from build123d import *

# Parameters (mm, degrees)
F0_W     = 58
F0_H     = 36
F0_R     = 1.25
F0_R_2   = 1.5
F1_DEPTH = 10
F0_R_3   = 1
F0_W_2   = 3.2825097442
F0_H_2   = 9.0816104785
F0_R_4   = 4
F2_DEPTH = 2.5
F3_R     = 3
F4_DEPTH = 6
F5_START = 0.9
F5_DEPTH = 16.2
F6_START = 6
F6_DEPTH = 10.7
F7_R     = 1


with BuildPart() as f1:
    # F0 (on Top) → F1 (new body)
    with BuildSketch(Plane.XY):
        with Locations((22.1260370687, 12.181818096)):
            Rectangle(F0_W, F0_H)
        with Locations((-2.8739629313, -1.818181904)):
            Circle(F0_R, mode=Mode.SUBTRACT)
        with Locations((3.1260370687, -3.018181904)):
            Circle(F0_R_2, mode=Mode.SUBTRACT)
        with Locations((41.1260370687, -3.018181904)):
            Circle(F0_R_2, mode=Mode.SUBTRACT)
        with Locations((47.1260370687, -1.818181904)):
            Circle(F0_R, mode=Mode.SUBTRACT)
        with BuildLine():
            Line((-0.0042433119, 0.0237876128), (-0.0123524841, 0.02397218))
            Line((-0.0123524841, 0.02397218), (-0.0123524841, 0.0693824727))
            ThreePointArc((-0.0123524841, 0.0693824727), (-1.0671188126, 12.0466773263), (-0.0123524841, 24.02397218))
            ThreePointArc((-0.0123524841, 24.02397218), (22.4498159336, 26.0118318189), (44.9770614896, 25))
            ThreePointArc((44.9770614896, 25), (46.474513746, 12), (44.9770614896, -1))
            ThreePointArc((44.9770614896, -1), (22.4574664967, -1.8971785964), (0, 0))
            ThreePointArc((0, 0), (-0.0021227043, 0.0118936194), (-0.0042433119, 0.0237876128))
        make_face(mode=Mode.SUBTRACT)
        with Locations((-2.8739629313, 26.181818096)):
            Circle(F0_R, mode=Mode.SUBTRACT)
        with Locations((3.1260370687, 27.16396598)):
            Circle(F0_R_2, mode=Mode.SUBTRACT)
        with Locations((41.1260370687, 27.6376707083)):
            Circle(F0_R_2, mode=Mode.SUBTRACT)
        with Locations((47.1260370687, 26.181818096)):
            Circle(F0_R, mode=Mode.SUBTRACT)
        with Locations((-2.8739629313, 26.181818096)):
            Circle(F0_R)
        with Locations((47.1260370687, 26.181818096)):
            Circle(F0_R)
        with Locations((47.1260370687, -1.818181904)):
            Circle(F0_R)
        with Locations((-2.8739629313, -1.818181904)):
            Circle(F0_R)
        with Locations((3.1260370687, -3.018181904)):
            Circle(F0_R_2)
        with Locations((3.1260370687, 27.16396598)):
            Circle(F0_R_2)
        with Locations((41.1260370687, 27.6376707083)):
            Circle(F0_R_2)
        with Locations((41.1260370687, -3.018181904)):
            Circle(F0_R_2)
    extrude(amount=F1_DEPTH)

    # F0 (on Top) → F2 (join)
    with BuildSketch(Plane.XY):
        with BuildLine():
            ThreePointArc((-0.0123524841, 24.02397218), (-1.0671188126, 12.0466773263), (-0.0123524841, 0.0693824727))
            Line((-0.0123524841, 0.0693824727), (-0.0123524841, 24.02397218))
        make_face()
        with BuildLine():
            Line((-0.0123524841, 24.02397218), (-0.0123524841, 0.0693824727))
            ThreePointArc((-0.0123524841, 0.0693824727), (-0.0083017494, 0.0465843578), (-0.0042433119, 0.0237876128))
            Line((-0.0042433119, 0.0237876128), (44.9770614896, -1))
            Line((44.9770614896, -1), (44.9770614896, 25))
            Line((44.9770614896, 25), (-0.0123524841, 24.02397218))
        make_face()
        with Locations((2.9621722015, 2.0848012064)):
            Circle(F0_R_3, mode=Mode.SUBTRACT)
        with Locations((5.0146379508, 11.9371688925)):
            Rectangle(F0_W_2, F0_H_2, mode=Mode.SUBTRACT)
        with Locations((41.7125664489, 2.0848012064)):
            Circle(F0_R_3, mode=Mode.SUBTRACT)
        with BuildLine():
            Line((26.1260370687, 7.1930042468), (26.1260370687, 9.181818096))
            Line((26.1260370687, 9.181818096), (26.4652403515, 9.181818096))
            ThreePointArc((26.4652403515, 9.181818096), (32.1260370687, 13.1930042468), (37.7868337859, 9.181818096))
            Line((37.7868337859, 9.181818096), (38.1260370687, 9.181818096))
            Line((38.1260370687, 9.181818096), (38.1260370687, 7.1930042468))
            Line((38.1260370687, 7.1930042468), (38.1260370687, 1.181818096))
            Line((38.1260370687, 1.181818096), (26.1260370687, 1.181818096))
            Line((26.1260370687, 1.181818096), (26.1260370687, 7.1930042468))
        make_face(mode=Mode.SUBTRACT)
        with Locations((41.1260370687, 12.181818096)):
            Circle(F0_R_2, mode=Mode.SUBTRACT)
        with Locations((18.8074270263, 12.2937392443)):
            Circle(F0_R_3, mode=Mode.SUBTRACT)
        with Locations((2.9621722015, 21.6664075851)):
            Circle(F0_R_3, mode=Mode.SUBTRACT)
        with Locations((26.8074270263, 12.2937392443)):
            Circle(F0_R_3, mode=Mode.SUBTRACT)
        with Locations((32.1260370687, 19.181818096)):
            Circle(F0_R_4, mode=Mode.SUBTRACT)
        with Locations((41.7125664489, 21.6664075851)):
            Circle(F0_R_3, mode=Mode.SUBTRACT)
        with BuildLine():
            Line((44.9770614896, -1), (-0.0042433119, 0.0237876128))
            ThreePointArc((-0.0042433119, 0.0237876128), (-0.0021227043, 0.0118936194), (0, 0))
            ThreePointArc((0, 0), (22.4574664967, -1.8971785964), (44.9770614896, -1))
        make_face()
        with BuildLine():
            ThreePointArc((44.9770614896, 25), (22.4498159336, 26.0118318189), (-0.0123524841, 24.02397218))
            Line((-0.0123524841, 24.02397218), (44.9770614896, 25))
        make_face()
        with BuildLine():
            Line((44.9770614896, 25), (44.9770614896, -1))
            ThreePointArc((44.9770614896, -1), (46.474513746, 12), (44.9770614896, 25))
        make_face()
        with Locations((2.9621722015, 21.6664075851)):
            Circle(F0_R_3)
        with Locations((2.9621722015, 2.0848012064)):
            Circle(F0_R_3)
        with Locations((41.7125664489, 2.0848012064)):
            Circle(F0_R_3)
        with Locations((41.7125664489, 21.6664075851)):
            Circle(F0_R_3)
        with Locations((18.8074270263, 12.2937392443)):
            Circle(F0_R_3)
        with Locations((26.8074270263, 12.2937392443)):
            Circle(F0_R_3)
        with Locations((5.0146379508, 11.9371688925)):
            Rectangle(F0_W_2, F0_H_2)
        with BuildLine():
            Line((26.4652403515, 9.181818096), (26.1260370687, 9.181818096))
            Line((26.1260370687, 9.181818096), (26.1260370687, 7.1930042468))
            ThreePointArc((26.1260370687, 7.1930042468), (26.2114457767, 8.2017707453), (26.4652403515, 9.181818096))
        make_face()
        with BuildLine():
            ThreePointArc((38.1260370687, 7.1930042468), (32.1260370687, 1.1930042468), (26.1260370687, 7.1930042468))
            Line((26.1260370687, 7.1930042468), (26.1260370687, 1.181818096))
            Line((26.1260370687, 1.181818096), (38.1260370687, 1.181818096))
            Line((38.1260370687, 1.181818096), (38.1260370687, 7.1930042468))
        make_face()
        with BuildLine():
            Line((38.1260370687, 9.181818096), (37.7868337859, 9.181818096))
            ThreePointArc((37.7868337859, 9.181818096), (38.0406283607, 8.2017707453), (38.1260370687, 7.1930042468))
            Line((38.1260370687, 7.1930042468), (38.1260370687, 9.181818096))
        make_face()
    extrude(amount=F2_DEPTH)

    # F3
    f3_edges = [f1.edges().sort_by_distance(p)[0] for p in [
        (51.126037, 30.181818, 5),
        (51.126037, -5.818182, 5),
        (-6.873963, -5.818182, 5),
        (-6.873963, 30.181818, 5),
    ]]
    fillet(f3_edges, radius=F3_R)

    # F0 (on Top) → F4 (join)
    with BuildSketch(Plane.XY):
        with Locations((5.0146379508, 11.9371688925)):
            Rectangle(F0_W_2, F0_H_2)
    extrude(amount=F4_DEPTH)

    # F0 (on Top) → F5 (cut)
    with BuildSketch(Plane.XY.offset(F5_START)):
        with Locations((47.1260370687, 26.181818096)):
            Circle(F0_R)
        with Locations((-2.8739629313, 26.181818096)):
            Circle(F0_R)
        with Locations((-2.8739629313, -1.818181904)):
            Circle(F0_R)
        with Locations((47.1260370687, -1.818181904)):
            Circle(F0_R)
    extrude(amount=F5_DEPTH, mode=Mode.SUBTRACT)

    # F0 (on Top) → F6 (cut)
    with BuildSketch(Plane.XY.offset(F6_START)):
        with Locations((3.1260370687, 27.16396598)):
            Circle(F0_R_2)
        with Locations((41.1260370687, 27.6376707083)):
            Circle(F0_R_2)
        with Locations((41.1260370687, -3.018181904)):
            Circle(F0_R_2)
        with Locations((3.1260370687, -3.018181904)):
            Circle(F0_R_2)
    extrude(amount=F6_DEPTH, mode=Mode.SUBTRACT)

    # F7
    f7_edges = [f1.edges().sort_by_distance(p)[0] for p in [
        (51.126037, 12.181818, 0),
        (22.126037, -5.818182, 0),
        (50.247357, -4.939502, 0),
        (50.247357, 29.303138, 0),
        (22.126037, 30.181818, 0),
        (-5.995283, 29.303138, 0),
        (-6.873963, 12.181818, 0),
        (-5.995283, -4.939502, 0),
    ]]
    fillet(f7_edges, radius=F7_R)


solid = f1.part
Part model, mm, in its own coordinate system. A direction names the side the tool comes from. Round coordinates to 2 decimals unless told otherwise and drop trailing zeros. Write each loop counter-clockwise with the first axis right and the second up, starting at its lowest first coordinate (ties: lowest second). Pieces come first, ordered by that corner, then holes. Notation, with made-up numbers: M -18.75,71 L 3.25,71 A22 cw 3.25,98 Z; hole C 24,21.5 d1. An arc over 180 degrees is marked long. Return JSON: item names as keys, results as strings. Group by question number.
(1) Saw through at D-D on x = 12. Write the cut outline in (y, z), then the cut area to 3 significant figures.
(2) Saw through at C-C on x = 27.5. Write the cut outline in (y, z), then the cut area to 3 significant figures.
(3) Which spindle directions (+Z, -Z, +X, -X, +Y, -Y) get a long thin tool onto all of the face, cutting with end or side? Do faces 1 (the face through (39.936, 11.269, 1.232)), 2 (the face through (5, 16.478, 4)). Say none if no direction does.
(4) Saw through at B-B on y = 20.5. Write the cut outline in (x, z), then the cut area to 3 significant figures.
(5) Two-plate mould, pull along Y, no slides. Class faces 3 (the face through (22, 12, 0)), 4 (the face through (3, -3, 6)), 5 (the face through (22, -5.818, 5)): +Y half, -Y half, draft (parallel to the pull), parting line (faces both ways), or undercut.
(6) Saw through at A-A on z = 5. Count the separate pieces of the cut face and the enclosed holes in it, then the cut area to 3 significant figures.
(7) Drill centre lines: probe 1 along Y at (x, z) = (-3, 1.5); probe 2 along X at (y, z) = (11, 8.75); probe 3 along Y at (x, z) = (-3.5, 4). Where is each one in solid material? Low to high.
(8) Pin check, flat tips, straight feed: pin 1 Ø1.5 at (x, y) = (47.13, 26.18) entering from +Z; pin 2 Ø1.5 at (x, y) = (3.5, -2.5) entering from +Z; pin 3 Ø12 at (x, y) = (15, 15) entering from +Z. Stop position of each tip, or through.
Returned:
{
 "1": {"outline": "M -5.82,1 A1 ccw -4.82,0 L 29.18,0 A1 ccw 30.18,1 L 30.18,10 L 25.46,10 L 25.46,2.5 L -1.36,2.5 L -1.36,10 L -5.82,10 Z", "area": "158 mm²"},
 "2": {"outline": "M -5.82,1 A1 ccw -4.82,0 L 3.37,0 L 3.37,2.5 L -1.94,2.5 L -1.94,10 L -5.82,10 Z; M 11.01,0 L 29.18,0 A1 ccw 30.18,1 L 30.18,10 L 26.05,10 L 26.05,2.5 L 11.01,2.5 Z", "area": "131 mm²"},
 "3": {"face 1": "+Z, -Z", "face 2": "+Z"},
 "4": {"outline": "M -6.87,1 A1 ccw -5.87,0 L 28.35,0 L 28.35,2.5 L -0.54,2.5 L -0.54,10 L -6.87,10 Z; M 35.9,0 L 50.13,0 A1 ccw 51.13,1 L 51.13,10 L 45.84,10 L 45.84,2.5 L 35.9,2.5 Z", "area": "213 mm²"},
 "5": {"face 3": "draft", "face 4": "undercut", "face 5": "-Y half"},
 "6": {"separate pieces": "2", "enclosed holes": "5", "area": "835 mm²"},
 "7": {"probe 1": "-5.82 to -3.06, -0.57 to 24.94, 27.43 to 30.18", "probe 2": "-6.87 to -1.06, 46.47 to 51.13", "probe 3": "-5.82 to -2.9, -0.74 to 25.1, 27.26 to 30.18"},
 "8": {"pin 1": "z = 0.9", "pin 2": "z = 6", "pin 3": "z = 2.5"}
}
